Model file for the job. Use its own axes, mm. A direction names the side the tool comes from. Give positions to 0.01 mm unless a question says otherwise; leave off trailing zeros.
```python
from build123d import *

# Parameters (mm, degrees)
SKETCH1_W           = 38.1
SKETCH1_H           = 4.826
SKETCH2_W           = 63.5
SKETCH2_H           = 4.826
BOSS_EXTRUDE1_DEPTH = 22.86
BOSS_EXTRUDE2_REACH = 601.968
SKETCH7_R           = 6.86435
SKETCH7_R_2         = 7.398290426
SKETCH7_R_3         = 6.940009574
BOSS_EXTRUDE3_DEPTH = 14.5542
BOSS_EXTRUDE4_REACH = 615.571
SKETCH9_R           = 2.06375
CUT_EXTRUDE1_DEPTH  = 10.16
BOSS_EXTRUDE5_DEPTH = 3.048


with BuildPart() as part:
    # Sketch1 → Loft1 section 0
    with BuildSketch(Plane.XY):
        with Locations((0, -2.413)):
            Rectangle(SKETCH1_W, SKETCH1_H)
    # Sketch2 → Loft1 section 1
    with BuildSketch(Plane.XY.offset(598.4875)):
        with Locations((0, -2.413)):
            Rectangle(SKETCH2_W, SKETCH2_H)
    loft()

    # Sketch5 → Boss-Extrude1 (add)
    with BuildSketch(Plane.XZ.offset(4.826)):
        Polygon((28.785543767, 458.7875), (31.75, 598.4875), (-31.75, 598.4875), (-28.785543767, 458.7875), align=None)
    extrude(amount=BOSS_EXTRUDE1_DEPTH)

    # Sketch4 for Loft2 → Loft2 section 0
    with BuildSketch(Plane.XY.offset(458.7875)):
        with BuildLine():
            Line((-28.785543767, -4.826), (28.785543767, -4.826))
            # circular arc as an exact rational Bezier (weights 1, cos(half-angle), 1)
            Bezier((28.785543767, -4.826), (0, -41.073048554), (-28.785543767, -4.826), weights=[1, 0.62189702, 1])
        make_face()
    # Sketch3 for Loft2 → Loft2 section 1
    with BuildSketch(Plane(origin=(0, 0, 0), x_dir=(-1, 0, 0), z_dir=(0, 0, -1))):
        with BuildLine():
            Line((19.05, -4.826), (-19.05, -4.826))
            Bezier((-19.05, -4.826), (0, -34.080271737), (19.05, -4.826), weights=[1, 0.545687389, 1])
        make_face()
    loft()

    # Boss-Extrude2: up to this face of the body (flat: up to its plane)
    boss_extrude2_end = Plane(part.part.faces().sort_by_distance((0, -27.686, 529.777696624))[0])
    # Sketch6 → Boss-Extrude2 (add, up to the picked face)
    with BuildSketch(Plane(origin=(0, 0, 0), x_dir=(1, 0, 0), z_dir=(0, 1, 0)), mode=Mode.PRIVATE) as boss_extrude2_sk1:
        with BuildLine():
            Line((-31.75, -598.4875), (-31.75, -601.5355))
            ThreePointArc((-31.75, -601.5355), (0, -608.5205), (31.75, -601.5355))
            Line((31.75, -601.5355), (31.75, -598.4875))
            Line((31.75, -598.4875), (-31.75, -598.4875))
        make_face()
    boss_extrude2_tool1 = split(extrude(boss_extrude2_sk1.sketch, amount=-BOSS_EXTRUDE2_REACH, mode=Mode.PRIVATE), bisect_by=boss_extrude2_end, keep=Keep.BOTH, mode=Mode.PRIVATE)
    add(boss_extrude2_tool1.solids().sort_by(Axis((0, 0, 602.638041), (0, -1, 0)))[0])

    # Sketch7 → Boss-Extrude3 (add)
    with BuildSketch(Plane(origin=(0, -23.749, 0), x_dir=(1, 0, 0), z_dir=(0, 1, 0))):
        with BuildLine():
            Line((-53.796563594, 36.394925453), (-17.858265722, 210.524988182))
            ThreePointArc((-17.858265722, 210.524988182), (27.686421042, 217.987818984), (32.564596867, 172.094292899))
            Line((32.564596867, 172.094292899), (29.99757559, 159.656431275))
            Line((29.99757559, 159.656431275), (29.99757559, 121.556431275))
            Line((29.99757559, 121.556431275), (54.47665, 32.656431275))
            ThreePointArc((54.47665, 32.656431275), (32.112450528, 21.373620039), (19.05, 0))
            Line((19.05, 0), (-19.05, 0))
            Line((-19.05, 0), (-19.05, 5.909460242))
            ThreePointArc((-19.05, 5.909460242), (-21.903905083, 13.930957291), (-29.182978723, 18.347321866))
            Line((-29.182978723, 18.347321866), (-43.925723247, 21.390042553))
            ThreePointArc((-43.925723247, 21.390042553), (-51.96875642, 26.848166031), (-53.796563594, 36.394925453))
        make_face()
        with Locations(Location((-21.72335, 44.196, 0), (0, 0, 180))):
            Circle(SKETCH7_R, mode=Mode.SUBTRACT)
        with Locations(Location((-12.122690426, 90.713602472, 0), (0, 0, 180))):
            Circle(SKETCH7_R_2, mode=Mode.SUBTRACT)
        with Locations(Location((-2.368009574, 137.977476641, 0), (0, 0, 180))):
            Circle(SKETCH7_R_3, mode=Mode.SUBTRACT)
        with Locations(Location((7.23265, 184.495079113, 0), (0, 0, 180))):
            Circle(SKETCH7_R, mode=Mode.SUBTRACT)
    extrude(amount=BOSS_EXTRUDE3_DEPTH)

    # Boss-Extrude4: up to this plane
    boss_extrude4_end = Plane(origin=(19.041425738, 0, -0.404062085), z_dir=(-0.999774928431425, 0, 0.021215383096688065))
    # Sketch8 → Boss-Extrude4 (add, up to the surface)
    with BuildSketch(Plane.ZY.offset(19.05), mode=Mode.PRIVATE) as boss_extrude4_sk1:
        Polygon((0, 0), (-2.286, 0), (-17.399, -9.1948), (0, -9.1948), align=None)
    boss_extrude4_tool1 = split(extrude(boss_extrude4_sk1.sketch, amount=-BOSS_EXTRUDE4_REACH, mode=Mode.PRIVATE), bisect_by=boss_extrude4_end, keep=Keep.BOTH, mode=Mode.PRIVATE)
    add(boss_extrude4_tool1.solids().sort_by_distance((-19.05, -5.773939, -5.888157))[0])

    # Sketch9 → Cut-Extrude1 (cut)
    with BuildSketch(Plane.XZ.offset(27.686)):
        with Locations((-18.459938241, 572.290233936)):
            Circle(SKETCH9_R)
        with Locations((18.968052603, 572.290233936)):
            Circle(SKETCH9_R)
        with Locations((19.026588432, 521.172733936)):
            Circle(SKETCH9_R)
        with Locations((-18.137388298, 521.172733936)):
            Circle(SKETCH9_R)
    extrude(amount=-CUT_EXTRUDE1_DEPTH, mode=Mode.SUBTRACT)

    # Sketch10 → Boss-Extrude5 (add)
    with BuildSketch(Plane.XY):
        with BuildLine():
            Line((-19.05, 0), (19.001490716, 0))
            Line((19.001490716, 0), (19.001490716, 1.6637))
            Line((19.001490716, 1.6637), (14.9098, 1.75792886))
            ThreePointArc((14.9098, 1.75792886), (14.286161326, 1.162367534), (13.6906, 1.786006208))
            Line((13.6906, 1.786006208), (5.505740514, 1.974497966))
            ThreePointArc((5.505740514, 1.974497966), (4.635244864, 1.143193615), (3.803940514, 2.013689264))
            Line((3.803940514, 2.013689264), (-4.283815101, 2.199944786))
            ThreePointArc((-4.283815101, 2.199944786), (-5.342420922, 1.188999326), (-6.353366381, 2.247605147))
            Line((-6.353366381, 2.247605147), (-13.5382, 2.413066988))
            ThreePointArc((-13.5382, 2.413066988), (-14.837447238, 1.172314226), (-16.0782, 2.471561463))
            Line((-16.0782, 2.471561463), (-19.05, 2.54))
            Line((-19.05, 2.54), (-19.05, 0))
        make_face()
    extrude(amount=BOSS_EXTRUDE5_DEPTH)


solid = part.part
```
1. Probe probe 1 along Y at (x, z) = (22, -111.5); probe 2 along Z at (x, y) = (-5, 0.5); probe 3 along Z at (x, y) = (4, -14). List the from-to ranges inside material, lowest first.
Calculated:
probe 1: y = -23.75 to -9.19
probe 2: z = 0 to 3.05
probe 3: z = -224.17 to -190.55, -178.44 to -140.74, -135.22 to 608.41
2. Pin check, flat tips, straight feed: P1, Ø0.8, axis at x = -8.5, y = 0.5, coming from the +Z side; P2, Ø4.5, axis at x = 18.97, z = 572.29, coming from the +Y side; P3, Ø2.5, axis at x = -18.46, z = 572.29, coming from the -Y side; P4, Ø12.5, axis at x = -2.37, z = -137.98, coming from the -Y side. Stop position of each tip, or through.
Calculated:
P1: stops at z = 3.05
P2: stops at y = 0
P3: stops at y = -17.53
P4: passes through
3. Which spindle directions (+Z, -Z, +X, -X, +Y, -Y) get a long thin tool onto all of the face, cutting with end or side? Do faces 4 (the flat face through (-19.05, -12, -5)), 5 (the flat face through (1, -23.749, -114)), 6 (the flat face through (0, -27.686, 535)), 7 (the flat face through (0, -23, 458.788)), 8 (the flat face through (42.066, -16.574, -77.729)). Say none if no direction does.
Calculated:
face 4: -X, +Y
face 5: -Z, +X, -X, -Y
face 6: +Z, -Z, +X, -X, -Y
face 7: -Y
face 8: +X, +Y, -Y
4. Pull direction Z, two halves, no side cores. Call faces 1 (the cylindrical face through (-0.46, -13.65, 608.52)), 2 (the cylindrical face through (-51.89, -16.57, -26.73)), 3 (the cylindrical face through (-14.866, -16.574, -43.894)): +Z half, -Z half, draft (parallel to the pull), parting line (faces both ways), or undercut.
Calculated:
face 1: +Z half
face 2: parting line
face 3: undercut
